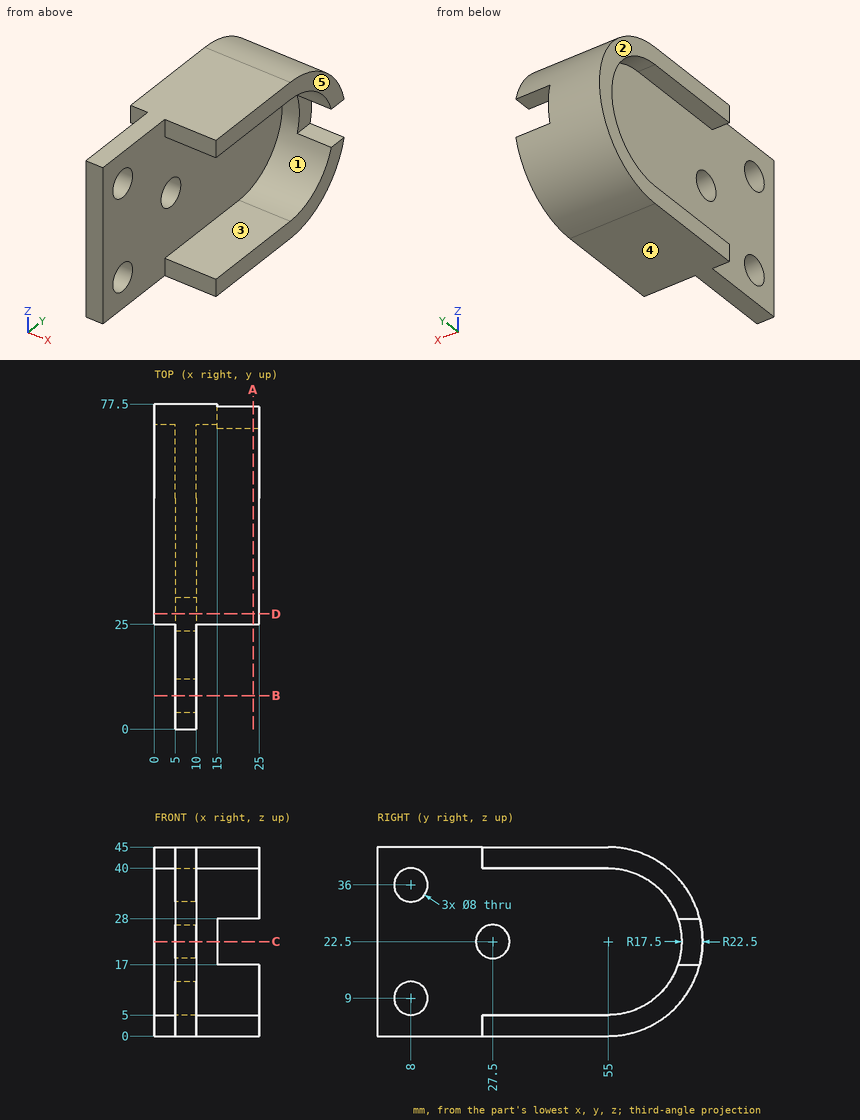
Check sheet for the drawn part. Datum: minimum x, y, z corner. Units: mm. A direction names the side the tool comes from. Round coordinates to 2 decimals unless told otherwise and drop trailing zeros. Order: outer loops, then holes, each group sorted by start corner. A loop starts at its lowest first (then second) coordinate and runs counter-clockwise, first axis right, second up. Notation, with made-up numbers: (65, 40) -> (113, 40) arc R24 ccw to (113, 71) -> close; hole circle Ø5 at (44, -35). An arc over 180 degrees is marked (long way). Return JSON: item names as keys, results as strings. Group by question number.
Q1. Section check A-A, the plane x = 23.5. Record the boundary of the cut face in (y, z), plus the area to 3 significant figures.
Q2. Section check D-D, the plane y = 27.5. Record the boundary of the cut face in (x, z).
Q3. Section check C-C, the plane z = 22.5. Record the boundary of the cut face in (x, y), plus the area to 4 significant figures.
Q4. Release check for a two-part mould opening along Z. For the marked faces 3, 4 and 5 record: released by +Z, released by -Z, zero draft, split by the parting line, or undercut.
Q5. Section check B-B, the plane y = 8. Record the boundary of the cut face in (x, z).
Q6. Tool access check on the marked faces 1 and 2. Record the directions out of +Z, -Z, +X, -X, +Y, -Y that give a thin tool (end or side, any length) a straight path to the whole face; none if there is none.
Q7. Material ranges on probe 1 along Z at (x, y) = (4.75, 51); probe 2 along Y at (x, z) = (6.2, 22.5); probe 3 along X at (y, z) = (42, 18.5), recorded low to high. Write a range as from..to.
Q8. Gauge pin test, flat ends, axial feed: pin 1 (3 mm diameter, centred on x = 12, z = 39.5, fed in from +Y); pin 2 (4.5 mm diameter, centred on y = 76, z = 23.5, fed in from +X); pin 3 (5.5 mm diameter, centred on x = 19.5, y = 73.5, fed in from +Z). Record the tip position at first contact, or that the pin passes through.
Numbers:
{
 "1": {"outline": "(25, 0) -> (55, 0) arc R22.5 ccw to (76.82, 17) -> (71.61, 17) arc R17.5 cw to (55, 5) -> (25, 5) -> close; (25, 40) -> (55, 40) arc R17.5 cw to (71.61, 28) -> (76.82, 28) arc R22.5 ccw to (55, 45) -> (25, 45) -> close", "area": "558 mm^2"},
 "2": {"outline": "(0, 0) -> (25, 0) -> (25, 5) -> (10, 5) -> (10, 18.5) -> (5, 18.5) -> (5, 5) -> (0, 5) -> close; (0, 40) -> (5, 40) -> (5, 26.5) -> (10, 26.5) -> (10, 40) -> (25, 40) -> (25, 45) -> (0, 45) -> close"},
 "3": {"outline": "(0, 72.5) -> (5, 72.5) -> (5, 31.5) -> (10, 31.5) -> (10, 72.5) -> (15, 72.5) -> (15, 77.5) -> (0, 77.5) -> close; (5, 0) -> (10, 0) -> (10, 23.5) -> (5, 23.5) -> close", "area": "397.5 mm^2"},
 "4": {"face 3": "undercut", "face 4": "released by -Z", "face 5": "zero draft"},
 "5": {"outline": "(5, 0) -> (10, 0) -> (10, 5) -> (5, 5) -> close; (5, 13) -> (10, 13) -> (10, 32) -> (5, 32) -> close; (5, 40) -> (10, 40) -> (10, 45) -> (5, 45) -> close"},
 "6": {"face 1": "+X, -Y", "face 2": "+Z, -Z, -X, +Y, -Y"},
 "7": {"probe 1": "0..5, 40..45", "probe 2": "0..23.5, 31.5..77.5", "probe 3": "5..10"},
 "8": {"pin 1": "y = 71.31", "pin 2": "x = 15", "pin 3": "z = 38.57"}
}
